Work out the finished part from the listing and answer in its coordinate system (mm). Face numbers are marked on the shaded views. A direction names the side the tool comes from. Coordinates: 2 decimals unless noted, no trailing zeros. Order: outer loops, then holes, each group sorted by start corner. A loop starts at its lowest first (then second) coordinate and runs counter-clockwise, first axis right, second up. Notation, with made-up numbers: (29, 14) -> (44, 14) arc R6 cw to (44, 25) -> close; hole circle Ø6 at (-12, -8). An arc over 180 degrees is marked (long way). Answer as CSV lines item,"result". Start each with the question number.
Item 1: Straight lines are drawn through the part: L1, parallel to Y at x = 0, z = 6.3; L2, parallel to X at y = 14, z = 0; L3, parallel to X at y = 6, z = -2. For each, find the intervals that lie inside material, in ascending order.
Item 2: Section A-A (x = 0) is taken. Write down the section's boundary in (y, z).
Item 3: Section D-D (y = 13) is taken. Write down the section's boundary in (x, z) (1 decimal).
Item 4: Which of the six approach directions +Z, -Z, +X, -X, +Y, -Y give full straight-line access (tool end or side, diameter ignored) to the marked faces 4, 5 and 6?
Item 5: Each of these flat-tipped pins is pushed along its axis until it touches: pin 1 Ø1.5 at (x, y) = (1, 12.5) entering from +Z; pin 2 Ø5.5 at (x, z) = (0, 0) entering from +Y; pin 3 Ø3 at (y, z) = (13, -4) entering from +X; pin 4 Ø4 at (y, z) = (14.5, -6) entering from -X. Where does it stop, or does it pass through?
Item 6: For a pull along X with two mould halves and no side action, classify the marked faces 1, 2 and 3 as pulls with the +X half, pulls with the -X half, needs draft (parallel to the pull), parting line crosses it, or undercut.
Item 7: Section C-C (z = 3.5) is taken. Write down the section's boundary in (x, y).
Item 8: Section B-B (z = -2.5) is taken. Write down the section's boundary in (x, y).
```python
from build123d import *

# Parameters (mm, degrees)
SKETCH2_R           = 7.9375
BOSS_EXTRUDE1_DEPTH = 20
SKETCH3_R           = 4
CUT_EXTRUDE1_DEPTH  = 8
SKETCH4_R           = 3
CUT_EXTRUDE2_DEPTH  = 12
SKETCH6_R           = 1.397
CUT_EXTRUDE3_DEPTH  = 6


with BuildPart() as part:
    # Sketch2 → Boss-Extrude1 (new body)
    with BuildSketch(Plane(origin=(0, 0, 0), x_dir=(1, 0, 0), z_dir=(0, 1, 0))):
        Circle(SKETCH2_R)
    extrude(amount=BOSS_EXTRUDE1_DEPTH)

    # Sketch3 → Cut-Extrude1 (cut)
    with BuildSketch(Plane(origin=(0, 20, 0), x_dir=(1, 0, 0), z_dir=(0, 1, 0))):
        Circle(SKETCH3_R)
    extrude(amount=-CUT_EXTRUDE1_DEPTH, mode=Mode.SUBTRACT)

    # Sketch4 → Cut-Extrude2 (cut)
    with BuildSketch(Plane.XZ):
        Circle(SKETCH4_R)
    extrude(amount=-CUT_EXTRUDE2_DEPTH, mode=Mode.SUBTRACT)

    # Sketch6 → Cut-Extrude3 (cut)
    with BuildSketch(Plane.XY.offset(7.9375)):
        with Locations((0, 6)):
            Circle(SKETCH6_R)
        with Locations((0, 16)):
            Circle(SKETCH6_R)
    extrude(amount=-CUT_EXTRUDE3_DEPTH, mode=Mode.SUBTRACT)


solid = part.part
```
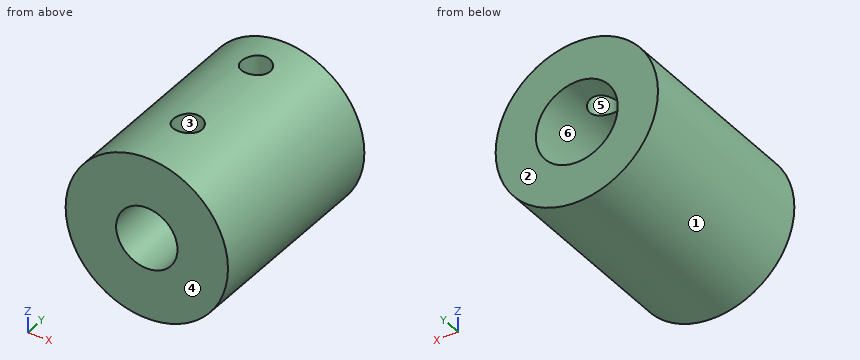
Checked values:
1,L1,"y = 0 to 4.6, 7.4 to 14.6, 17.4 to 20"
1,L2,"x = -7.94 to -4, 4 to 7.94"
1,L3,"x = -7.68 to -2.24, 2.24 to 7.68"
2,outline,"(0, -7.94) -> (20, -7.94) -> (20, -4) -> (12, -4) -> (12, -3) -> (0, -3) -> close; (0, 3) -> (4.6, 3) -> (4.6, 7.94) -> (0, 7.94) -> close; (7.4, 3) -> (12, 3) -> (12, 4) -> (14.6, 4) -> (14.6, 7.94) -> (7.4, 7.94) -> close; (17.4, 4) -> (20, 4) -> (20, 7.94) -> (17.4, 7.94) -> close"
3,outline,"circle Ø15.9 at (0, 0); hole circle Ø8 at (0, 0)"
4,face 4,"+Z, -Z, +X, -X, -Y"
4,face 5,"+Z"
4,face 6,"+Y"
5,pin 1,"stops at z = 7.93"
5,pin 2,"passes through"
5,pin 3,"stops at x = 7.53"
5,pin 4,"stops at x = -6.86"
6,face 1,"parting line crosses it"
6,face 2,"needs draft"
6,face 3,"undercut"
7,outline,"(-7.12, 0) -> (7.12, 0) -> (7.12, 20) -> (1.94, 20) -> (1.94, 12) -> (-1.94, 12) -> (-1.94, 20) -> (-7.12, 20) -> close; hole circle Ø2.79 at (0, 6)"
8,outline,"(-7.53, 0) -> (-1.66, 0) -> (-1.66, 12) -> (-3.12, 12) -> (-3.12, 20) -> (-7.53, 20) -> close; (1.66, 0) -> (7.53, 0) -> (7.53, 20) -> (3.12, 20) -> (3.12, 12) -> (1.66, 12) -> close"
